from build123d import *

# Parameters (mm, degrees)
SKETCH1_W                                   = 80
SKETCH1_H                                   = 24
BOSS_EXTRUDE1_DEPTH                         = 65
F_2_MM_TOP_BOT_3_MM_SIDE_T                  = -3
F_2_MM_TOP_BOT_3_MM_SIDE_THICKNESS_2_FACE_W = 59
F_2_MM_TOP_BOT_3_MM_SIDE_THICKNESS_2_FACE_H = 21
F_2_MM_TOP_BOT_3_MM_SIDE_THICKNESS_2_DEPTH  = 2
F_2_MM_TOP_BOT_3_MM_SIDE_THICKNESS_3_FACE_W = 21
F_2_MM_TOP_BOT_3_MM_SIDE_THICKNESS_3_FACE_H = 59
F_2_MM_TOP_BOT_3_MM_SIDE_THICKNESS_3_DEPTH  = 2
F_9_8_MM_PORT_HOLES_DEPTH                   = 3
SKETCH4_R                                   = 3.55
F_7_1_MM_FIXTURE_HOLES_DEPTH                = 10
F_2_MM_RADIUS_R                             = 2
F_8_5_START                                 = -2
SKETCH7_R                                   = 4.25
F_8_5_MM_HOLD_OFFSET_2_MM_DEPTH             = 3.2
R2_FILET_R                                  = 2
SKETCH8_W                                   = 3
SKETCH8_H                                   = 3
F_7_MM_NOTCH_DEPTH                          = 7


with BuildPart() as part:
    # Sketch1 → Boss-Extrude1 (new body)
    with BuildSketch(Plane(origin=(0, 0, 0), x_dir=(0, 1, 0), z_dir=(0, 0, 1))):
        Rectangle(SKETCH1_W, SKETCH1_H)
    extrude(amount=BOSS_EXTRUDE1_DEPTH)

    # 2 mm top/bot 3 mm side
    f_2_mm_top_bot_3_mm_side_openings = [part.faces().sort_by_distance(p)[0] for p in [
        (-12, 0, 32.5),
    ]]
    offset(amount=F_2_MM_TOP_BOT_3_MM_SIDE_T, openings=f_2_mm_top_bot_3_mm_side_openings, kind=Kind.INTERSECTION)

    # 2 mm top/bot 3 mm side thickness 2 face (on inner face of the shell) → 2 mm top/bot 3 mm side thickness 2 (add)
    with BuildSketch(Plane(origin=(-1.5, 37, 32.5), x_dir=(0, 0, 1), z_dir=(0, 1, 0))):
        Rectangle(F_2_MM_TOP_BOT_3_MM_SIDE_THICKNESS_2_FACE_W, F_2_MM_TOP_BOT_3_MM_SIDE_THICKNESS_2_FACE_H)
    extrude(amount=-F_2_MM_TOP_BOT_3_MM_SIDE_THICKNESS_2_DEPTH)

    # 2 mm top/bot 3 mm side thickness 3 face (on inner face of the shell) → 2 mm top/bot 3 mm side thickness 3 (add)
    with BuildSketch(Plane(origin=(-1.5, -37, 32.5), x_dir=(-1, 0, 0), z_dir=(0, -1, 0))):
        Rectangle(F_2_MM_TOP_BOT_3_MM_SIDE_THICKNESS_3_FACE_W, F_2_MM_TOP_BOT_3_MM_SIDE_THICKNESS_3_FACE_H)
    extrude(amount=-F_2_MM_TOP_BOT_3_MM_SIDE_THICKNESS_3_DEPTH)

    # Sketch3 → 9.8 mm port holes (cut)
    with BuildSketch(Plane(origin=(0, 0, 0), x_dir=(1, 0, 0), z_dir=(0, 0, -1))):
        with BuildLine():
            ThreePointArc((4.9, 22.5), (3.464823228, 25.964823228), (0, 27.4))
            Line((0, 27.4), (0, 17.6))
            ThreePointArc((0, 17.6), (3.464823228, 19.035176772), (4.9, 22.5))
        make_face()
        with BuildLine():
            Line((0, 17.6), (0, 27.4))
            ThreePointArc((0, 27.4), (-4.9, 22.5), (0, 17.6))
        make_face()
        with BuildLine():
            ThreePointArc((4.9, 7.5), (3.464823228, 10.964823228), (0, 12.4))
            Line((0, 12.4), (0, 2.6))
            ThreePointArc((0, 2.6), (3.464823228, 4.035176772), (4.9, 7.5))
        make_face()
        with BuildLine():
            Line((0, 2.6), (0, 12.4))
            ThreePointArc((0, 12.4), (-4.9, 7.5), (0, 2.6))
        make_face()
        with BuildLine():
            ThreePointArc((4.9, -7.5), (3.464823228, -4.035176772), (0, -2.6))
            Line((0, -2.6), (0, -12.4))
            ThreePointArc((0, -12.4), (3.464823228, -10.964823228), (4.9, -7.5))
        make_face()
        with BuildLine():
            Line((0, -12.4), (0, -2.6))
            ThreePointArc((0, -2.6), (-4.9, -7.5), (0, -12.4))
        make_face()
        with BuildLine():
            ThreePointArc((4.9, -22.5), (3.464823228, -19.035176772), (0, -17.6))
            Line((0, -17.6), (0, -27.4))
            ThreePointArc((0, -27.4), (3.464823228, -25.964823228), (4.9, -22.5))
        make_face()
        with BuildLine():
            Line((0, -27.4), (0, -17.6))
            ThreePointArc((0, -17.6), (-4.9, -22.5), (0, -27.4))
        make_face()
    extrude(amount=-F_9_8_MM_PORT_HOLES_DEPTH, mode=Mode.SUBTRACT)

    # Sketch4 → 7.1 mm fixture holes (cut)
    with BuildSketch(Plane.XY.offset(65)):
        with Locations((0, 24.2)):
            Circle(SKETCH4_R)
        Circle(SKETCH4_R)
        with Locations((0, -24.2)):
            Circle(SKETCH4_R)
        with BuildLine():
            ThreePointArc((0, -3.55), (-3.55, 0), (0, 3.55))
            Line((0, 3.55), (-12, 3.55))
            Line((-12, 3.55), (-12, -3.55))
            Line((-12, -3.55), (0, -3.55))
        make_face()
    extrude(amount=-F_7_1_MM_FIXTURE_HOLES_DEPTH, mode=Mode.SUBTRACT)

    # 2 mm radius
    f_2_mm_radius_edges = [part.edges().sort_by_distance(p)[0] for p in [
        (9, -35, 32.5),
        (9, 35, 32.5),
        (12, -40, 32.5),
        (12, 40, 32.5),
    ]]
    fillet(f_2_mm_radius_edges, radius=F_2_MM_RADIUS_R)

    # Sketch7 → 8.5 mm hold offset 2 mm (cut)
    with BuildSketch(Plane(origin=(0, 40, 0), x_dir=(-1, 0, 0), z_dir=(0, 1, 0)).offset(F_8_5_START)):
        with Locations(Location((1, 32.5, 0), (0, 0, 90))):
            Circle(SKETCH7_R)
    f_8_5_mm_hold_offset_2_mm = extrude(amount=-F_8_5_MM_HOLD_OFFSET_2_MM_DEPTH, mode=Mode.SUBTRACT)

    # magnet slot mirror: 8.5 mm hold offset 2 mm across plane
    add(f_8_5_mm_hold_offset_2_mm.mirror(Plane.ZX), mode=Mode.SUBTRACT)

    # R2 filet
    r2_filet_edges = [part.edges().sort_by_distance(p)[0] for p in [
        (9, 0, 3),
        (9, 0, 62),
        (-2.5, 35, 3),
        (-2.5, -35, 3),
        (8.414213562, -34.414213562, 3),
        (8.414213562, 34.414213562, 3),
        (-2.5, 35, 62),
        (-2.5, -35, 62),
        (8.414213562, -34.414213562, 62),
        (8.414213562, 34.414213562, 62),
        (12, 0, 0),
        (12, 0, 65),
        (-1, -40, 0),
        (-1, 40, 0),
        (11.414213562, 39.414213562, 0),
        (11.414213562, -39.414213562, 0),
        (-1, -40, 65),
        (-1, 40, 65),
        (11.414213562, 39.414213562, 65),
        (11.414213562, -39.414213562, 65),
    ]]
    fillet(r2_filet_edges, radius=R2_FILET_R)

    # Sketch8 → 7 mm notch (cut)
    with BuildSketch(Plane(origin=(-12, 0, 0), x_dir=(0, -1, 0), z_dir=(-1, 0, 0))):
        with Locations((-35, 32.5)):
            Rectangle(SKETCH8_W, SKETCH8_H)
    f_7_mm_notch = extrude(amount=-F_7_MM_NOTCH_DEPTH, mode=Mode.SUBTRACT)

    # 7 mm notch mirror: 7 mm notch across plane
    add(f_7_mm_notch.mirror(Plane.ZX), mode=Mode.SUBTRACT)


solid = part.part
Geometry check sheet. Reference: the model listing, model coordinates, mm. A direction names the side the tool comes from. Round coordinates to 2 decimals unless told otherwise and drop trailing zeros. Write each loop counter-clockwise with the first axis right and the second up, starting at its lowest first coordinate (ties: lowest second). Pieces come first, ordered by that corner, then holes. Notation, with made-up numbers: (-38, -25) - (-18, -25) arc R22 cw to (-18, 12) - close; hole circle Ø2 at (-30, 36). An arc over 180 degrees is marked (long way). One line per item, written item: value.
1. Scan lines: L1, parallel to Y at x = -7.5, z = 45.5; L2, parallel to Z at x = -1, y = -36.7; L3, parallel to Z at x = -8, y = 19. Record each from-to range of solid material in increasing order.
The answers:
L1: y = -40 to -35, 35 to 40
L2: z = 0 to 28.25, 36.75 to 65
L3: z = 0 to 3, 62 to 65
2. Mould release check, pull along Y, two halves, no side actions. Record for faces 1 (the face through (-1, 40, 32)), 2 (the face through (-0.85, -39.4, 0.57)), 3 (the face through (4, 0, 62)): released by +Y, released by -Y, zero draft, split by the parting line, or undercut.
The answers:
face 1: released by +Y
face 2: released by -Y
face 3: undercut
3. Set-up check for faces 4 (the face through (-2.63, 34.43, 3.6)), 5 (the face through (-0.46, -20.68, 63.52)), 6 (the face through (3.214, 36.521, 31.947)), 7 (the face through (3.55, -0.08, 63.52)): record each of +Z, -Z, +X, -X, +Y, -Y from which the full face is reachable in a straight line by a thin tool's end or side.
The answers:
face 4: -X
face 5: +Z
face 6: none
face 7: +Z, -X
4. Cross-section at A-A on y = 0. Record the boundary of the cut face in (x, z), and give its area (3 significant figures).
The answers:
outline: (-12, 0) - (10, 0) arc R2 ccw to (12, 2) - (12, 63) arc R2 ccw to (10, 65) - (3.55, 65) - (3.55, 62) - (7, 62) arc R2 cw to (9, 60) - (9, 5) arc R2 cw to (7, 3) - (-12, 3) - close
area: 274 mm^2
5. Depth check by flat-ended pin: pin 1 Ø8 at (x, y) = (0, -24.2) entering from +Z; pin 2 Ø1.5 at (x, z) = (-9, 64) entering from +Y; pin 3 Ø3 at (y, z) = (21, 16) entering from -X. Enter the tip coordinate at first touch or a pass-through.
The answers:
pin 1: stops at z = 65
pin 2: stops at y = 39.98
pin 3: stops at x = 9
6. Cross-section at B-B on z = 32.5. Record the boundary of the cut face in (x, y).
The answers:
outline: (-12, -40) - (10, -40) arc R2 ccw to (12, -38) - (12, 38) arc R2 ccw to (10, 40) - (-12, 40) - (-12, 36.5) - (-5.25, 36.5) - (-5.25, 38) - (3.25, 38) - (3.25, 35) - (7, 35) arc R2 cw to (9, 33) - (9, -33) arc R2 cw to (7, -35) - (3.25, -35) - (3.25, -38) - (-5.25, -38) - (-5.25, -36.5) - (-12, -36.5) - close
7. Cross-section at C-C on x = -7.5. Record the boundary of the cut face in (y, z), and give its area (3 significant figures).
The answers:
outline: (-40, 2) arc R2 ccw to (-38, 0) - (38, 0) arc R2 ccw to (40, 2) - (40, 63) arc R2 ccw to (38, 65) - (3.55, 65) - (3.55, 62) - (33, 62) arc R2 cw to (35, 60) - (35, 34) - (36.5, 34) - (36.5, 31) - (35, 31) - (35, 5) arc R2 cw to (33, 3) - (-33, 3) arc R2 cw to (-35, 5) - (-35, 31) - (-36.5, 31) - (-36.5, 34) - (-35, 34) - (-35, 60) arc R2 cw to (-33, 62) - (-3.55, 62) - (-3.55, 65) - (-38, 65) arc R2 ccw to (-40, 63) - close
area: 1,040 mm^2
8. Cross-section at D-D on y = -24.2. Record the boundary of the cut face in (x, z).
The answers:
outline: (-12, 0) - (-4.6, 0) - (-4.6, 3) - (-12, 3) - close; (-12, 62) - (-3.55, 62) - (-3.55, 65) - (-12, 65) - close; (3.55, 62) - (7, 62) arc R2 cw to (9, 60) - (9, 5) arc R2 cw to (7, 3) - (4.6, 3) - (4.6, 0) - (10, 0) arc R2 ccw to (12, 2) - (12, 63) arc R2 ccw to (10, 65) - (3.55, 65) - close
